Can you work these out from the model? Positions are in its coordinate system, mm. Face numbers are marked on the shaded views. A direction names the side the tool comes from. Coordinates: 2 decimals unless noted, no trailing zeros. Order: outer loops, then holes, each group sorted by start corner. A loop starts at its lowest first (then second) coordinate and runs counter-clockwise, first axis right, second up.
```python
from build123d import *

# Parameters (mm, degrees)
CROQUIS1_R                 = 0.5
SALIENTE_EXTRUIR1_DEPTH    = 6
CORTAR_EXTRUIR6_DEPTH      = 9.883720712
CORTAR_EXTRUIR6_DEPTH_BACK = 9.883720712
CROQUIS3_W                 = 6
CROQUIS3_H                 = 4
CORTAR_EXTRUIR2_DEPTH      = 9.509571903
CORTAR_EXTRUIR7_DEPTH      = 9.509571903
CORTAR_EXTRUIR7_DEPTH_BACK = 9.509571903
CORTAR_EXTRUIR1_DEPTH      = 9.509571933
CORTAR_EXTRUIR1_DEPTH_BACK = 9.509571933
CROQUIS2_R                 = 0.5


with BuildPart() as part:
    # Croquis1 → Saliente-Extruir1 (new body)
    with BuildSketch(Plane.XY):
        with BuildLine():
            ThreePointArc((-4.615384615, 1.902971827), (-6, 0), (-4.615384615, -1.902971827))
            ThreePointArc((-4.615384615, -1.902971827), (0, -2.630683123), (4.615384615, -1.902971827))
            ThreePointArc((4.615384615, -1.902971827), (6, 0), (4.615384615, 1.902971827))
            ThreePointArc((4.615384615, 1.902971827), (0, 2.630683123), (-4.615384615, 1.902971827))
        make_face()
        with Locations((4, 0)):
            Circle(CROQUIS1_R, mode=Mode.SUBTRACT)
    extrude(amount=SALIENTE_EXTRUIR1_DEPTH)

    # Croquis7 → Cortar-Extruir6 (cut, two sides: drawn at the far end of the back side and taken through both)
    with BuildSketch(Plane(origin=(0, 0, 0), x_dir=(1, 0, 0), z_dir=(0, 1, 0)).offset(-CORTAR_EXTRUIR6_DEPTH_BACK)):
        Polygon((-6, 0), (6, 0), (6, -3), (6, -6), (-6, -6), (-6, -3), align=None)
        with BuildLine():
            Line((-2.441311123, -5.430683123), (2.441311123, -5.430683123))
            ThreePointArc((2.441311123, -5.430683123), (3.538199894, -5.207416005), (4.615384615, -4.902971827))
            ThreePointArc((4.615384615, -4.902971827), (6, -3), (4.615384615, -1.097028173))
            ThreePointArc((4.615384615, -1.097028173), (3.538199894, -0.792583995), (2.441311123, -0.569316877))
            Line((2.441311123, -0.569316877), (-2.441311123, -0.569316877))
            ThreePointArc((-2.441311123, -0.569316877), (-3.538199894, -0.792583995), (-4.615384615, -1.097028173))
            ThreePointArc((-4.615384615, -1.097028173), (-6, -3), (-4.615384615, -4.902971827))
            ThreePointArc((-4.615384615, -4.902971827), (-3.538199894, -5.207416005), (-2.441311123, -5.430683123))
        make_face(mode=Mode.SUBTRACT)
    extrude(amount=CORTAR_EXTRUIR6_DEPTH + CORTAR_EXTRUIR6_DEPTH_BACK, mode=Mode.SUBTRACT)

    # Croquis3 → Cortar-Extruir2 (cut, through all)
    with BuildSketch(Plane.XY):
        with Locations((-3, 0)):
            Rectangle(CROQUIS3_W, CROQUIS3_H)
    extrude(amount=CORTAR_EXTRUIR2_DEPTH, mode=Mode.SUBTRACT)

    # Croquis4 → Cortar-Extruir7 (cut, two sides: drawn at the far end of the back side and taken through both)
    with BuildSketch(Plane(origin=(0, 0, 0), x_dir=(1, 0, 0), z_dir=(0, 1, 0)).offset(-CORTAR_EXTRUIR7_DEPTH_BACK)):
        with BuildLine():
            ThreePointArc((-2.164743401, -0.526342579), (-3.242933174, -0.724065618), (-4.303804421, -1))
            Line((-4.303804421, -1), (-4.303804421, -3))
            ThreePointArc((-4.303804421, -3), (-3.694875017, -1.364872858), (-2.164743401, -0.526342579))
        make_face()
        with BuildLine():
            ThreePointArc((-2.164743401, -5.473657421), (-3.694875017, -4.635127142), (-4.303804421, -3))
            Line((-4.303804421, -3), (-4.303804421, -5))
            ThreePointArc((-4.303804421, -5), (-3.242933174, -5.275934382), (-2.164743401, -5.473657421))
        make_face()
    extrude(amount=CORTAR_EXTRUIR7_DEPTH + CORTAR_EXTRUIR7_DEPTH_BACK, mode=Mode.SUBTRACT)

    # Croquis2 → Cortar-Extruir1 (cut, two sides: drawn at the far end of the back side and taken through both)
    with BuildSketch(Plane(origin=(0, 0, 0), x_dir=(1, 0, 0), z_dir=(0, 1, 0)).offset(-CORTAR_EXTRUIR1_DEPTH_BACK)):
        with Locations(Location((-2.803804421, -3, 0), (0, 0, 270))):
            Circle(CROQUIS2_R)
    extrude(amount=CORTAR_EXTRUIR1_DEPTH + CORTAR_EXTRUIR1_DEPTH_BACK, mode=Mode.SUBTRACT)


solid = part.part
```
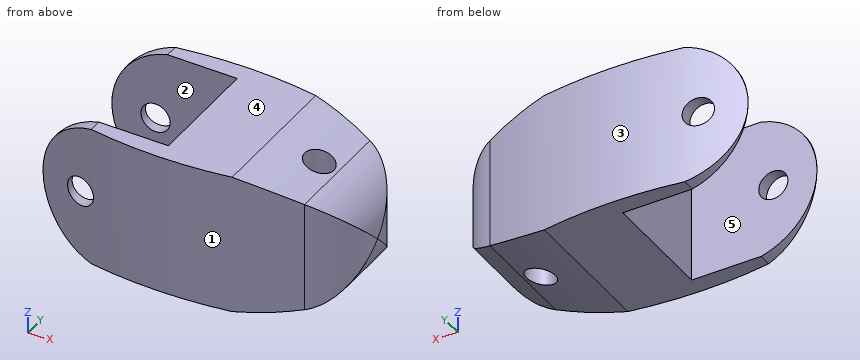
1. I'm going to push flat-ended pins straight in: pin 1 (1.3 mm diameter, centred on x = -2, z = 3, fed in from +Y); pin 2 (1.2 mm diameter, centred on y = -1, z = 2.5, fed in from -X); pin 3 (1.3 mm diameter, centred on x = -2.5, z = 2.5, fed in from -Y). Where does each tip first touch, or does it pass through?
Completed:
pin 1: stops at y = 2.57
pin 2: stops at x = 0
pin 3: stops at y = -2.52
2. On a 3-axis mill with a long thin cutter (end or side, diameter ignored), from which of +Z, -Z, +X, -X, +Y, -Y can I reach the whole of each face in a straight line? I mean the marked faces 1 and 2. Say none if no direction works.
Completed:
face 1: +Z, -Z, -Y
face 2: +Z, -Z, -X
3. Thinking about a two-plate mould opening in Y: for the marked faces 3, 4 and 5, which applies, pulls with the +Y half, pulls with the -Y half, needs draft (parallel to the pull), parting line crosses it, or undercut?
Completed:
face 3: pulls with the +Y half
face 4: needs draft
face 5: undercut
4. Imagine slicing it at D-D on x = 4. Please give me the cut outline in (y, z), then the cut area to 3 significant figures.
Completed:
outline: (-2.09, 0.91) - (-0.5, 0.91) - (-0.5, 5.09) - (-2.09, 5.09) - close; (0.5, 0.91) - (2.09, 0.91) - (2.09, 5.09) - (0.5, 5.09) - close
area: 13.3 mm2
5. Imagine slicing it at B-B on y = -0.3. Please give me the cut outline in (x, z), then the cut area to 3 significant figures.
Completed:
outline: (0, 0.57) - (2.44, 0.57) arc R15 ccw to (3.6, 0.81) - (3.6, 5.19) arc R15 ccw to (2.44, 5.43) - (0, 5.43) - close; (4.4, 1.03) arc R15 ccw to (4.62, 1.1) arc R2 ccw to (5.98, 2.7) - (5.98, 3.3) arc R2 ccw to (4.62, 4.9) arc R15 ccw to (4.4, 4.97) - close
area: 21.9 mm2
6. Imagine slicing it at C-C on z = 4.6. Please give me the cut outline in (x, y).
Completed:
outline: (-3.72, -2.16) arc R15 ccw to (4.62, -1.9) arc R2 ccw to (5.2, -1.6) - (5.2, 1.6) arc R2 ccw to (4.62, 1.9) arc R15 ccw to (-3.72, 2.16) - (-3.72, 2) - (0, 2) - (0, -2) - (-3.72, -2) - close; hole circle Ø1 at (4, 0)
7. Imagine slicing it at A-A on x = -0.25. Please give me the cut outline in (y, z), then the cut area to 3 significant figures.
Completed:
outline: (-2.63, 0.57) - (-2, 0.57) - (-2, 5.43) - (-2.63, 5.43) - close; (2, 0.57) - (2.63, 0.57) - (2.63, 5.43) - (2, 5.43) - close
area: 6.11 mm2
8. Please list where these lines run through material, in increasing order: probe 1 along Y at (x, z) = (-3, 1.9); probe 2 along Y at (x, z) = (-0.5, 4.2); probe 3 along X at (y, z) = (-0.15, 1).
Completed:
probe 1: y = -2.33 to -2, 2 to 2.33
probe 2: y = -2.62 to -2, 2 to 2.62
probe 3: x = 0 to 3.52
